Verification items for this drawing (mm, ordinates from the low corner). A direction names the side the tool comes from. Round coordinates to 2 decimals unless told otherwise and drop trailing zeros. Order: outer loops, then holes, each group sorted by start corner. A loop starts at its lowest first (then second) coordinate and runs counter-clockwise, first axis right, second up. Notation, with made-up numbers: (-1, 27) -> (10, 27) arc R6 cw to (10, 31) -> close; hole circle Ø3 at (-37, 87.5). An arc over 180 degrees is marked (long way). Put each result on its own line as item: value.
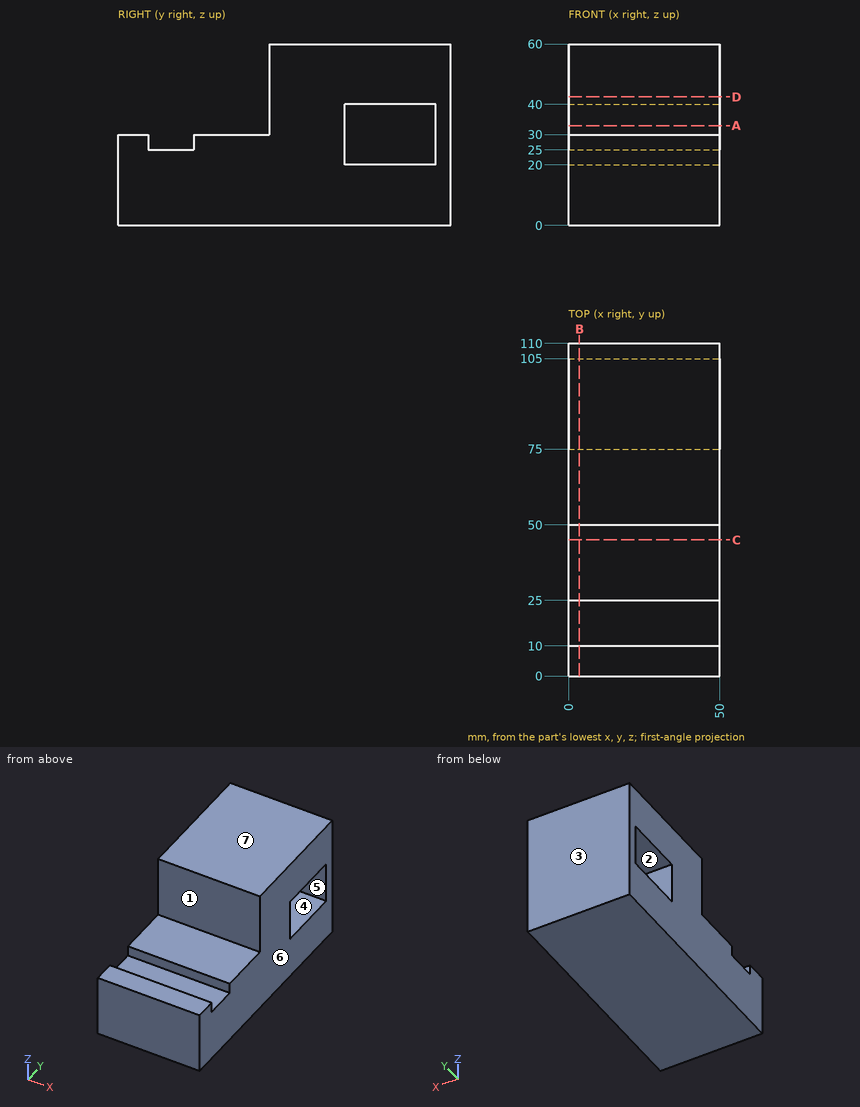
Item 1: Gauge pin test, flat ends, axial feed: pin 1 Ø8 at (x, y) = (16.5, 4) entering from +Z; pin 2 Ø9 at (x, z) = (17.5, 42.5) entering from -Y; pin 3 Ø4.5 at (x, y) = (26.5, 14) entering from +Z. Record the tip position at first contact, or that the pin passes through.
Check sheet entries:
pin 1: stops at z = 30
pin 2: stops at y = 50
pin 3: stops at z = 25
Item 2: Section check B-B on x = 3.5. Record the boundary of the cut face in (y, z), then the cut area to 4 significant figures.
Check sheet entries:
outline: (0, 0) -> (110, 0) -> (110, 60) -> (50, 60) -> (50, 30) -> (25, 30) -> (25, 25) -> (10, 25) -> (10, 30) -> (0, 30) -> close; hole (75, 20) -> (105, 20) -> (105, 40) -> (75, 40) -> close
area: 4,425 mm^2
Item 3: Section check D-D on z = 42.5. Record the boundary of the cut face in (x, y).
Check sheet entries:
outline: (0, 50) -> (50, 50) -> (50, 110) -> (0, 110) -> close
Item 4: Release check for a two-part mould opening along Z. For the marked faces 4, 5, 6 and 7 record: +Z half, -Z half, draft (parallel to the pull), parting line (faces both ways), or undercut.
Check sheet entries:
face 4: undercut
face 5: undercut
face 6: draft
face 7: +Z half
Item 5: Section check A-A on z = 33. Record the boundary of the cut face in (x, y).
Check sheet entries:
outline: (0, 50) -> (50, 50) -> (50, 75) -> (0, 75) -> close; (0, 105) -> (50, 105) -> (50, 110) -> (0, 110) -> close
Item 6: Section check C-C on y = 45. Record the boundary of the cut face in (x, z).
Check sheet entries:
outline: (0, 0) -> (50, 0) -> (50, 30) -> (0, 30) -> close
Item 7: Tool access check on the marked faces 1, 2 and 3. Record the directions out of +Z, -Z, +X, -X, +Y, -Y that give a thin tool (end or side, any length) a straight path to the whole face; none if there is none.
Check sheet entries:
face 1: +Z, +X, -X, -Y
face 2: +X, -X
face 3: +Z, -Z, +X, -X, +Y
Item 8: Material ranges on L1, parallel to Y at x = 35, z = 28; L2, parallel to Y at x = 5.5, z = 38; L3, parallel to Z at x = 28.5, y = 6.5, recorded low to high. Write a range as [from, to].
Check sheet entries:
L1: y = [0, 10], [25, 75], [105, 110]
L2: y = [50, 75], [105, 110]
L3: z = [0, 30]
